The listing builds one solid part. Answer for the finished solid, in the listing's coordinates (mm). A direction names the side the tool comes from. Coordinates: 2 decimals unless noted, no trailing zeros. Write each loop counter-clockwise with the first axis right and the second up, starting at its lowest first coordinate (ties: lowest second). Pieces come first, ordered by that corner, then holes.
from build123d import *

# Parameters (mm, degrees)
SKETCH_W        = 30
SKETCH_H        = 20
PAD_DEPTH       = 48
SKETCH001_W     = 24
SKETCH001_H     = 14
POCKET_DEPTH    = 30
SKETCH002_R     = 2
POCKET001_DEPTH = 18.001
SKETCH003_R     = 6
POCKET002_DEPTH = 14
SKETCH004_W     = 10
SKETCH004_H     = 31.196079
POCKET003_DEPTH = 20.001


with BuildPart() as part:
    # Sketch → Pad (new body)
    with BuildSketch(Plane.XY):
        Rectangle(SKETCH_W, SKETCH_H)
    extrude(amount=PAD_DEPTH)

    # Sketch001 (on Face6 of Pad) → Pocket (cut)
    with BuildSketch(Plane.XY.offset(48)):
        Rectangle(SKETCH001_W, SKETCH001_H)
    extrude(amount=-POCKET_DEPTH, mode=Mode.SUBTRACT)

    # Sketch002 (on Face11 of Pocket) → Pocket001 (cut, through all)
    with BuildSketch(Plane.XY.offset(18)):
        Circle(SKETCH002_R)
    extrude(amount=-POCKET001_DEPTH, mode=Mode.SUBTRACT)

    # Sketch003 (on Face12 of Pocket001) → Pocket002 (cut)
    with BuildSketch(Plane.XY.offset(18)):
        Circle(SKETCH003_R)
    extrude(amount=-POCKET002_DEPTH, mode=Mode.SUBTRACT)

    # Sketch004 (on Face6 of Pocket002) → Pocket003 (cut, through all)
    with BuildSketch(Plane.XZ.offset(10)):
        with Locations((0, 33.598039)):
            Rectangle(SKETCH004_W, SKETCH004_H)
    extrude(amount=-POCKET003_DEPTH, mode=Mode.SUBTRACT)


solid = part.part
1. Section D-D on y = -5 is taken. Give the vertices of the cut face in (x, z).
Results found:
outline: (-15, 0) - (15, 0) - (15, 48) - (12, 48) - (12, 18) - (3.32, 18) - (3.32, 4) - (-3.32, 4) - (-3.32, 18) - (-12, 18) - (-12, 48) - (-15, 48) - close
2. Section C-C on y = 0 is taken. Give the vertices of the cut face in (x, z), then the cut area to 3 significant figures.
Results found:
outline: (-15, 0) - (-2, 0) - (-2, 4) - (-6, 4) - (-6, 18) - (-12, 18) - (-12, 48) - (-15, 48) - close; (2, 0) - (15, 0) - (15, 48) - (12, 48) - (12, 18) - (6, 18) - (6, 4) - (2, 4) - close
area: 536 mm2
3. A tool of negligible diameter and unlimited length cuts with its end or side. For faces 5 (the flat face through (-5, 9, 33)), 6 (the cylindrical face through (0, -2, 2)), 7 (the flat face through (-12, 0, 33)), from which of +Z, -Z, +X, -X, +Y, -Y can it reach the whole face along a straight path? Write none if from no direction.
Results found:
face 5: +Z, +Y, -Y
face 6: +Z, -Z
face 7: +Z
4. Flat-ended cylindrical pins translate along their axes: P1, Ø10, axis at x = 0, y = -7, coming from the -Z side; P2, Ø5.5, axis at x = -7, y = 0.5, coming from the +Z side; P3, Ø3.5, axis at x = 0.5, y = -1, coming from the +Z side. Find the tip coordinate at first contact, or state that the pin passes through.
Results found:
P1: stops at z = 0
P2: stops at z = 18
P3: stops at z = 4
5. For a pull along X with two mould halves and no side action, classify faces 1 (the flat face through (-5, -8, 33)), 2 (the cylindrical face through (-6, 0, 11)), 3 (the flat face through (-15, 0, 24)), 4 (the flat face through (-0.2, 2.4, 0)) as pulls with the +X half, pulls with the -X half, needs draft (parallel to the pull), parting line crosses it, or undercut.
Results found:
face 1: undercut
face 2: undercut
face 3: pulls with the -X half
face 4: needs draft
6. Find the intervals of material crossed by L1, parallel to Y at x = -9.25, z = 20; L2, parallel to X at y = 0, z = 12; L3, parallel to X at y = 0.75, z = 31.5, in increasing order.
Results found:
L1: y = -10 to -7, 7 to 10
L2: x = -15 to -6, 6 to 15
L3: x = -15 to -12, 12 to 15
7. Section A-A on x = 0 is taken. Give the vertices of the cut face in (y, z), then the cut area to 3 significant figures.
Results found:
outline: (-10, 0) - (-2, 0) - (-2, 4) - (-6, 4) - (-6, 18) - (-10, 18) - close; (2, 0) - (10, 0) - (10, 18) - (6, 18) - (6, 4) - (2, 4) - close
area: 176 mm2
8. Section B-B on z = 37 is taken. Give the vertices of the cut face in (x, y).
Results found:
outline: (-15, -10) - (-5, -10) - (-5, -7) - (-12, -7) - (-12, 7) - (-5, 7) - (-5, 10) - (-15, 10) - close; (5, -10) - (15, -10) - (15, 10) - (5, 10) - (5, 7) - (12, 7) - (12, -7) - (5, -7) - close
